For this review, take the finished solid that the model builds, in its own axes (mm). Face numbers are marked on the shaded views. A direction names the side the tool comes from. Give positions to 0.01 mm unless a question says otherwise; leave off trailing zeros. Write each loop counter-clockwise with the first axis right and the second up, starting at its lowest first coordinate (ties: lowest second). Pieces come first, ordered by that corner, then holes. Notation, with made-up numbers: (52, 36) -> (99, 36) arc R32 ccw to (99, 75) -> close; hole circle Ø5 at (22, 82.25). An arc over 180 degrees is marked (long way). Write item = value, one per line.
Autodesk Inventor part; units mm, degrees
ref_plane "YZ Plane" through (0, 0, 0) normal (1, 0, 0) x (0, 1, 0)
ref_plane "XZ Plane" through (0, 0, 0) normal (0, 1, 0) x (-1, 0, 0)
ref_plane "XY Plane" through (0, 0, 0) normal (0, 0, 1) x (1, 0, 0)
sketch "Sketch1" plane through (0, 0, 0) normal (0, 1, 0) x (-1, 0, 0)
  line L0 (13, 6) -> (-13, 6)
  line L1 (-13, 6) -> (-13, -6)
  line L2 (-13, -6) -> (13, -6)
  line L3 (13, -6) -> (13, 6)
  point P0 (0, 0)
  dimension "d0" = 6
  dimension "d1" = 6
  dimension "d2" = 26
  dimension "d3" = 13
extrude "Extrusion1" add sketch "Sketch1" along normal blind 10
sketch "Sketch2" plane through (13, 0, 6) normal (1, 0, 0) x (0, 0, -1)
  line L0 (0, 10) -> (0, 0)
  circle A0 centre (6, 5) radius 1
  point P0 (6, 0)
  dimension "d6" = 2
extrude "Extrusion2" add sketch "Sketch2" along normal blind 5
sketch "Sketch3" plane through (18, 5, 0) normal (1, 0, 0) x (0, 0, -1)
  circle A0 centre (0, 0) radius 16
  point P0 (0, -5)
  dimension "d9" = 32
extrude "Extrusion3" add sketch "Sketch3" along normal blind 7
properties part number "Motor"
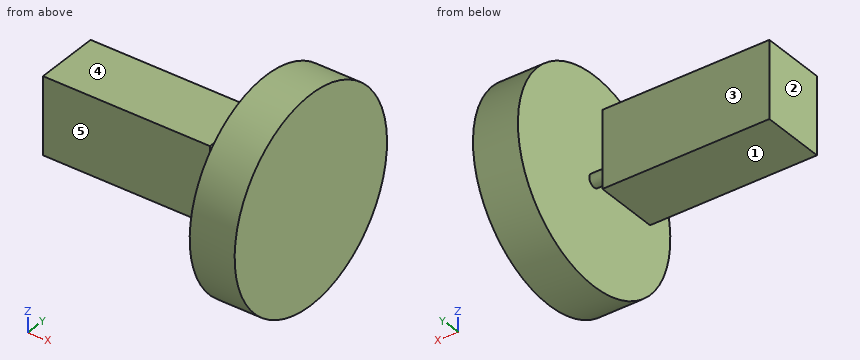
(1) To check wall thickness, follow probe 1 along X at (y, z) = (7.5, -1.5); probe 2 along Y at (x, z) = (8.5, -4.5); probe 3 along X at (y, z) = (9, -14). State the ranges of each line that lie inside material, in increasing order.
Answers below:
probe_1 = -13 to 13, 18 to 25
probe_2 = 0 to 10
probe_3 = 18 to 25
(2) Take a section at B-B (y = 5). Write out the cut boundary in (x, z).
Answers below:
outline = (-13, -6) -> (13, -6) -> (13, -1) -> (18, -1) -> (18, -16) -> (25, -16) -> (25, 16) -> (18, 16) -> (18, 1) -> (13, 1) -> (13, 6) -> (-13, 6) -> close
(3) Take a section at D-D (z = -5). Write out the cut boundary in (x, y).
Answers below:
outline = (-13, 0) -> (13, 0) -> (13, 10) -> (-13, 10) -> close; (18, -10.2) -> (25, -10.2) -> (25, 20.2) -> (18, 20.2) -> close
(4) For pin 1 (12 mm diameter, centred on x = 8, y = 1, fed in from +Z); pin 2 (9.5 mm diameter, centred on x = -5.5, z = -1, fed in from +Y); pin 3 (1 mm diameter, centred on y = 2, z = -9, fed in from -X), all flat-tipped, find the tip position at first contact; note any pin that passes through.
Answers below:
pin_1 = 6
pin_2 = 10
pin_3 = 18
(5) Take a section at A-A (z = 0). Write out the cut boundary in (x, y), plus the area to 3 significant figures.
Answers below:
outline = (-13, 0) -> (13, 0) -> (13, 4) -> (18, 4) -> (18, -11) -> (25, -11) -> (25, 21) -> (18, 21) -> (18, 6) -> (13, 6) -> (13, 10) -> (-13, 10) -> close
area = 494 mm^2
(6) Tool access review of the marked faces 1, 2, 3, 4 and 5: name each direction out of +Z, -Z, +X, -X, +Y, -Y from which nothing blocks a thin tool from reaching the whole face with its end or side.
Answers below:
face_1 = -Z, -X, +Y, -Y
face_2 = +Z, -Z, -X, +Y, -Y
face_3 = +Z, -Z, -X, +Y
face_4 = +Z, -X, +Y, -Y
face_5 = +Z, -Z, -X, -Y
(7) Take a section at C-C (y = 9). Write out the cut boundary in (x, z).
Answers below:
outline = (-13, -6) -> (13, -6) -> (13, 6) -> (-13, 6) -> close; (18, -15.49) -> (25, -15.49) -> (25, 15.49) -> (18, 15.49) -> close
